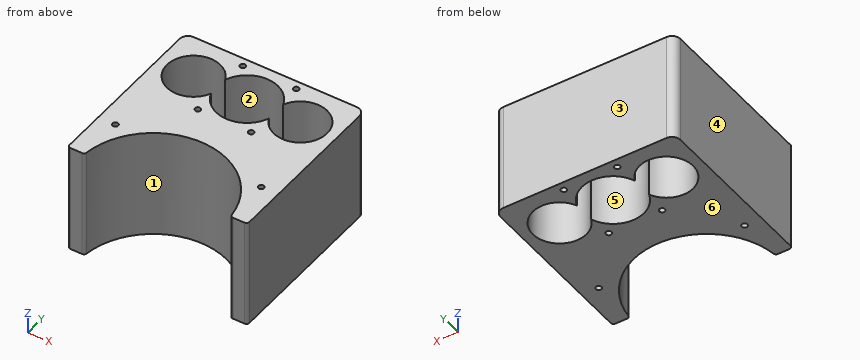
from build123d import *

# Parameters (mm, degrees)
SKETCH_1_R      = 1
EXTRUDE_1_DEPTH = 39


with BuildPart() as part:
    # Эскиз1 → Бобышка-Вытянуть1 (new body)
    with BuildSketch(Plane.XY):
        with BuildLine():
            Line((-32, -17), (-32, 12))
            ThreePointArc((-32, 12), (-31.121320344, 14.121320344), (-29, 15))
            Line((-29, 15), (29, 15))
            ThreePointArc((29, 15), (31.121320344, 14.121320344), (32, 12))
            Line((32, 12), (32, -17))
            Line((32, -17), (32, -46.753646645))
            ThreePointArc((32, -46.753646645), (31.707106781, -47.460753426), (31, -47.753646645))
            Line((31, -47.753646645), (26.804126359, -47.753646645))
            ThreePointArc((26.804126359, -47.753646645), (26.140890093, -47.50205673), (25.811380939, -46.873881955))
            ThreePointArc((25.811380939, -46.873881955), (0, -24), (-25.811380939, -46.873881955))
            ThreePointArc((-25.811380939, -46.873881955), (-26.140890093, -47.50205673), (-26.804126359, -47.753646645))
            Line((-26.804126359, -47.753646645), (-31, -47.753646645))
            ThreePointArc((-31, -47.753646645), (-31.707106781, -47.460753426), (-32, -46.753646645))
            Line((-32, -46.753646645), (-32, -17))
        make_face()
        with Locations((-9.5, 12)):
            Circle(SKETCH_1_R, mode=Mode.SUBTRACT)
        with Locations((9.5, 12)):
            Circle(SKETCH_1_R, mode=Mode.SUBTRACT)
        with Locations((9.5, -12)):
            Circle(SKETCH_1_R, mode=Mode.SUBTRACT)
        with Locations((-9.5, -12)):
            Circle(SKETCH_1_R, mode=Mode.SUBTRACT)
        with Locations((-25.902777778, -31.358962601)):
            Circle(SKETCH_1_R, mode=Mode.SUBTRACT)
        with Locations((26, -31.358962601)):
            Circle(SKETCH_1_R, mode=Mode.SUBTRACT)
        with BuildLine():
            ThreePointArc((-10.309210526, -3.836688458), (0, -11), (10.309210526, -3.836688458))
            ThreePointArc((10.309210526, -3.836688458), (28.5, 0), (10.309210526, 3.836688458))
            ThreePointArc((10.309210526, 3.836688458), (0, 11), (-10.309210526, 3.836688458))
            ThreePointArc((-10.309210526, 3.836688458), (-28.5, 0), (-10.309210526, -3.836688458))
        make_face(mode=Mode.SUBTRACT)
    extrude(amount=EXTRUDE_1_DEPTH)


solid = part.part
Model file for the job. Use its own axes, mm. Face numbers are marked on the shaded views. A direction names the side the tool comes from. Give positions to 0.01 mm unless a question says otherwise; leave off trailing zeros. Write each loop counter-clockwise with the first axis right and the second up, starting at its lowest first coordinate (ties: lowest second). Pieces come first, ordered by that corner, then holes. Notation, with made-up numbers: (-29, -4.5) -> (-12, -4.5) arc R24 cw to (-12, 13.5) -> close; hole circle Ø8 at (61, 74.25). An arc over 180 degrees is marked (long way). Write item = value, one per line.
(1) Tool access for the marked faces 5 and 6: list every direction of +Z, -Z, +X, -X, +Y, -Y with a clear straight run to the whole face (end or side of a thin tool).
Determined:
face_5 = +Z, -Z
face_6 = -Z, +X, -X, +Y, -Y
(2) Slice it at C-C, the plane z = 15. Give the cut face in (x, y), then the cut area to 3 significant figures.
Determined:
outline = (-32, -46.75) arc R1 ccw to (-31, -47.75) -> (-26.8, -47.75) arc R1 ccw to (-25.81, -46.87) arc R26 cw to (25.81, -46.87) arc R1 ccw to (26.8, -47.75) -> (31, -47.75) arc R1 ccw to (32, -46.75) -> (32, 12) arc R3 ccw to (29, 15) -> (-29, 15) arc R3 ccw to (-32, 12) -> close; hole circle Ø2 at (-25.9, -31.36); hole circle Ø2 at (-9.5, -12); hole circle Ø2 at (-9.5, 12); hole (-10.31, -3.84) arc R11 ccw to (10.31, -3.84) arc R9.5 ccw (long way) to (10.31, 3.84) arc R11 ccw to (-10.31, 3.84) arc R9.5 ccw (long way) to start; hole circle Ø2 at (9.5, -12); hole circle Ø2 at (9.5, 12); hole circle Ø2 at (26, -31.36)
area = 2,120 mm2
(3) Slice it at B-B, the plane y = -42. Give the cut face in (x, z).
Determined:
outline = (-32, 0) -> (-24.74, 0) -> (-24.74, 39) -> (-32, 39) -> close; (24.74, 0) -> (32, 0) -> (32, 39) -> (24.74, 39) -> close
(4) Mould opens along Y. For the marked faces 1, 2, 3 and 4 say: released by +Y, released by -Y, zero draft, split by the parting line, or undercut.
Determined:
face_1 = released by -Y
face_2 = undercut
face_3 = released by +Y
face_4 = zero draft
(5) Flat gauge pins, fed straight in: P1, Ø4, axis at x = 4.5, z = 14.5, coming from the -Y side; P2, Ø12, axis at x = -20.5, z = 15.5, coming from the -Y side. Where does each tip first touch, or does it go through?
Determined:
P1 = -24.83
P2 = -47.71
(6) Probe line 1 along Y through (x, z) = (-9.5, 15); line 2 along X through (y, z) = (8, 7); line 3 along Y through (x, z) = (26, 14). List the from-to ranges inside material, lowest first.
Determined:
line_1 = -25.8 to -13, -11 to -5.55, 5.55 to 11, 13 to 15
line_2 = -32 to -24.12, -13.88 to -7.55, 7.55 to 13.88, 24.12 to 32
line_3 = -47.35 to -32.36, -30.36 to -6.42, 6.42 to 15
(7) Slice it at A-A, the plane x = 15. Give the cut face in (y, z).
Determined:
outline = (-28.76, 0) -> (-8.62, 0) -> (-8.62, 39) -> (-28.76, 39) -> close; (8.62, 0) -> (15, 0) -> (15, 39) -> (8.62, 39) -> close
